CAD build for the part. Positions are in the model's coordinates, mm. Face numbers are marked on the shaded views. A direction names the side the tool comes from. Give positions to 0.01 mm unless a question says otherwise; leave off trailing zeros. Loops run counter-clockwise (first coordinate to the right, second up) from the corner with the lowest first, then second, coordinate; pieces in that order, holes last.
```python
from build123d import *

# Parameters (mm, degrees)
F2_DEPTH = 6.35
F1_R     = 11.0236
F3_DEPTH = 6.35
F4_SIZE  = 1.27


with BuildPart() as f2:
    # F0 (on Top) → F2 (new body)
    with BuildSketch(Plane.XY):
        Polygon((-6.4158048664, 17.4625), (6.4158048664, 17.4625), (12.8316097327, 28.575), (6.4158048664, 39.6875), (-6.4158048664, 39.6875), (-12.8316097327, 28.575), align=None)
        Polygon((10.0893114241, 28.575), (5.0446557121, 19.8374), (-5.0446557121, 19.8374), (-10.0893114241, 28.575), (-5.0446557121, 37.3126), (5.0446557121, 37.3126), align=None, mode=Mode.SUBTRACT)
    extrude(amount=F2_DEPTH)

    # F1 (on face) → F3 (join)
    with BuildSketch(Plane.XY):
        with BuildLine():
            Line((-6.4158048664, 17.4625), (-9.6237072152, 23.0187498538))
            Line((-9.6237072152, 23.0187498538), (-12.8316097327, 28.575))
            Line((-12.8316097327, 28.575), (-17.0211530549, 17.4625))
            Line((-17.0211530549, 17.4625), (-5.038242593, 13.3696958763))
            ThreePointArc((-5.038242593, 13.3696958763), (-0.124129265, 14.2869607746), (4.8051799463, 13.4552183904))
            Line((4.8051799463, 13.4552183904), (-6.4158048664, 17.4625))
        make_face()
        with BuildLine():
            ThreePointArc((5.038242593, 13.3696958763), (4.9218970272, 13.4129633528), (4.8051799463, 13.4552183904))
            ThreePointArc((4.8051799463, 13.4552183904), (-0.124129265, 14.2869607746), (-5.038242593, 13.3696958763))
            Line((-5.038242593, 13.3696958763), (5.038242593, 13.3696958763))
        make_face()
        with BuildLine():
            Line((5.038242593, 13.3696958763), (-5.038242593, 13.3696958763))
            ThreePointArc((-5.038242593, 13.3696958763), (-14.2875, 0), (-5.038242593, -13.3696958763))
            Line((-5.038242593, -13.3696958763), (5.038242593, -13.3696958763))
            ThreePointArc((5.038242593, -13.3696958763), (11.7498201539, -8.1286150482), (14.2875, 0))
            ThreePointArc((14.2875, 0), (11.7498201539, 8.1286150482), (5.038242593, 13.3696958763))
        make_face()
        Circle(F1_R, mode=Mode.SUBTRACT)
        with BuildLine():
            Line((5.038242593, -13.3696958763), (-5.038242593, -13.3696958763))
            ThreePointArc((-5.038242593, -13.3696958763), (-4.9218969503, -13.412963381), (-4.805179792, -13.4552184455))
            ThreePointArc((-4.805179792, -13.4552184455), (0.1241293469, -14.2869607739), (5.038242593, -13.3696958763))
        make_face()
        with BuildLine():
            ThreePointArc((5.038242593, -13.3696958763), (0.1241293469, -14.2869607739), (-4.805179792, -13.4552184455))
            Line((-4.805179792, -13.4552184455), (0, -15.1712628866))
            Line((0, -15.1712628866), (6.4158048664, -17.4625))
            Line((6.4158048664, -17.4625), (8.5332421601, -21.1300089747))
            Line((8.5332421601, -21.1300089747), (8.8309233846, -17.1881254571))
            Line((8.8309233846, -17.1881254571), (13.9178989278, -18.9255993827))
            Line((13.9178989278, -18.9255993827), (11.2879660769, -25.9013307593))
            Line((11.2879660769, -25.9013307593), (12.8316097327, -28.575))
            Line((12.8316097327, -28.575), (17.0211530549, -17.4625))
            Line((17.0211530549, -17.4625), (5.038242593, -13.3696958763))
        make_face()
        with BuildLine():
            Line((6.4158048664, -39.6875), (9.6237072578, -34.1312500723))
            ThreePointArc((9.6237072578, -34.1312500723), (5.5562499639, -38.1987073204), (0, -39.6875))
            Line((0, -39.6875), (6.4158048664, -39.6875))
        make_face()
        with BuildLine():
            ThreePointArc((9.6237071905, -23.0187498111), (5.5562499055, -18.9512926459), (0, -17.4625))
            ThreePointArc((0, -17.4625), (-5.556249932, -18.9512926612), (-9.623707221, -23.018749864))
            ThreePointArc((-9.623707221, -23.018749864), (-11.1125, -28.5750000026), (-9.6237072184, -34.1312501405))
            ThreePointArc((-9.6237072184, -34.1312501405), (-5.5562499298, -38.1987073401), (0, -39.6875))
            ThreePointArc((0, -39.6875), (5.5562499639, -38.1987073204), (9.6237072578, -34.1312500723))
            ThreePointArc((9.6237072578, -34.1312500723), (10.7338507338, -31.451126679), (11.1125, -28.575))
            ThreePointArc((11.1125, -28.575), (10.7338507164, -25.6988732559), (9.6237071905, -23.0187498111))
        make_face()
        Polygon((0, -19.8374), (5.0446557121, -19.8374), (7.5669837696, -24.2062003489), (10.0893114241, -28.575), (7.5669837791, -32.9437996345), (5.0446557121, -37.3126), (0, -37.3126), (-5.0446557121, -37.3126), (-7.5669835677, -32.9438000008), (-10.0893114241, -28.575), (-7.5669835463, -24.2061999623), (-5.0446557121, -19.8374), align=None, mode=Mode.SUBTRACT)
        with BuildLine():
            Line((9.6237072578, -34.1312500723), (12.8316097327, -28.575))
            Line((12.8316097327, -28.575), (11.2879660769, -25.9013307593))
            Line((11.2879660769, -25.9013307593), (9.6237071905, -23.0187498111))
            ThreePointArc((9.6237071905, -23.0187498111), (10.7338507164, -25.6988732559), (11.1125, -28.575))
            ThreePointArc((11.1125, -28.575), (10.7338507338, -31.451126679), (9.6237072578, -34.1312500723))
        make_face()
        with BuildLine():
            ThreePointArc((0, -39.6875), (-5.5562499298, -38.1987073401), (-9.6237072184, -34.1312501405))
            Line((-9.6237072184, -34.1312501405), (-6.4158048664, -39.6875))
            Line((-6.4158048664, -39.6875), (0, -39.6875))
        make_face()
        with BuildLine():
            ThreePointArc((-9.6237072184, -34.1312501405), (-11.1125, -28.5750000026), (-9.623707221, -23.018749864))
            Line((-9.623707221, -23.018749864), (-12.8316097327, -28.575))
            Line((-12.8316097327, -28.575), (-9.6237072184, -34.1312501405))
        make_face()
        with BuildLine():
            ThreePointArc((-9.623707221, -23.018749864), (-5.556249932, -18.9512926612), (0, -17.4625))
            Line((0, -17.4625), (-6.4158048664, -17.4625))
            Line((-6.4158048664, -17.4625), (-9.623707221, -23.018749864))
        make_face()
        with BuildLine():
            Line((8.5332421601, -21.1300089747), (6.4158048664, -17.4625))
            Line((6.4158048664, -17.4625), (0, -17.4625))
            ThreePointArc((0, -17.4625), (5.5562499055, -18.9512926459), (9.6237071905, -23.0187498111))
            Line((9.6237071905, -23.0187498111), (8.5332421601, -21.1300089747))
        make_face()
        Polygon((6.4158048664, -17.4625), (0, -15.1712628866), (0, -17.4625), align=None)
    extrude(amount=F3_DEPTH)

    # F4
    f4_edges = [f2.edges().sort_by_distance(p)[0] for p in [
        (-11.029698, 15.416098, 6.35),
        (-14.926381, 23.01875, 6.35),
        (-9.623707, 34.13125, 6.35),
        (0, 39.6875, 6.35),
        (9.623707, 34.13125, 6.35),
        (9.623707, 23.01875, 6.35),
        (0, 17.4625, 6.35),
        (-0.805312, 15.458859, 6.35),
        (14.286961, 0.124129, 6.35),
        (-14.286961, -0.124129, 6.35),
        (9.623707, -34.13125, 6.35),
        (0, -39.6875, 6.35),
        (-9.623707, -34.13125, 6.35),
        (-9.623707, -23.01875, 6.35),
        (-3.207902, -17.4625, 6.35),
        (14.926381, -23.01875, 6.35),
        (11.029698, -15.416098, 6.35),
        (-2.40259, -14.313241, 6.35),
    ]]
    chamfer(f4_edges, length=F4_SIZE)


solid = f2.part
```
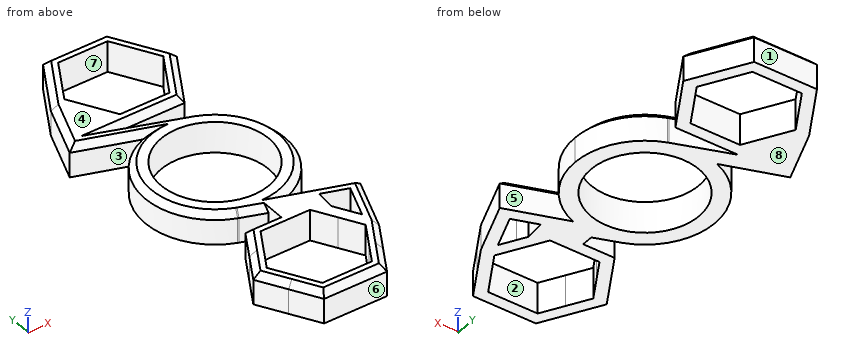
1. Drop flat-ended pins along their axis: pin 1 (1 mm diameter, centred on y = -13, z = 3, fed in from -X); pin 2 (10 mm diameter, centred on x = 13.5, y = -22.5, fed in from -Z). Give the stop position or say it passes through.
Responses:
pin 1: stops at x = -6.92
pin 2: stops at z = 0
2. Saw through at B-B, the plane z = 2. Count the separate pieces of the cut face and the enclosed holes in it, and give its area (3 significant figures).
Responses:
separate pieces: 1
enclosed holes: 4
area: 757 mm2
3. Tool access for the marked faces 1, 2, 3, 4 and 5: list every direction of +Z, -Z, +X, -X, +Y, -Y with a clear straight run to the whole face (end or side of a thin tool).
Responses:
face 1: +Z, -Z, +X, -X, +Y
face 2: +Z, -Z
face 3: +Z, -Z, -X
face 4: +Z, +X, -X, +Y, -Y
face 5: +Z, -Z, +X
4. Saw through at C-C, the plane y = 21. List the corners of the cut face in (x, z), and give its area (3 significant figures).
Responses:
outline: (-15.69, 0) - (-5.72, 0) - (-5.72, 6.35) - (-14.33, 6.35) - (-15.69, 5.08) - close; (5.72, 0) - (8.46, 0) - (8.46, 5.08) - (6.99, 6.35) - (5.72, 6.35) - close
area: 78.9 mm2
5. Pull direction Y, two halves, no side cores. Call the marked faces 6, 7 and 8: released by +Y, released by -Y, zero draft, split by the parting line, or undercut.
Responses:
face 6: released by -Y
face 7: undercut
face 8: zero draft
6. Probe line 1 along Y through (x, z) = (-2, 2); line 2 along Y through (x, z) = (-4.5, 1.5); line 3 along X through (y, z) = (34, 4.75). List the from-to ranges inside material, lowest first.
Responses:
line 1: y = -39.69 to -37.31, -19.84 to -17.46, -14.46 to -10.84, 10.84 to 15.89, 17.46 to 19.84, 37.31 to 39.69
line 2: y = -39.69 to -37.31, -19.84 to -17.46, -13.56 to -10.06, 10.06 to 16.78, 17.46 to 19.84, 37.31 to 39.69
line 3: x = -9.7 to -6.96, 6.96 to 9.7
7. Saw through at A-A, the plane y = 30. List the corners of the cut face in (x, z), and give its area (3 significant figures).
Responses:
outline: (-12.01, 0) - (-9.27, 0) - (-9.27, 6.35) - (-10.54, 6.35) - (-12.01, 5.08) - close; (9.27, 0) - (12.01, 0) - (12.01, 5.08) - (10.54, 6.35) - (9.27, 6.35) - close
area: 33.0 mm2
